The model under review builds one solid part; all positions refer to its coordinate system, in mm. A direction names the side the tool comes from. Coordinates: 2 decimals unless noted, no trailing zeros. Answer in a Markdown table with one row per item.
from build123d import *

# Parameters (mm, degrees)
SKETCH1_W                                        = 80
SKETCH1_H                                        = 50
BOSS_EXTRUDE1_DEPTH                              = 30
CBORE_FOR_M10_HEX_HEAD_BOLT8_D                   = 5
CBORE_FOR_M10_HEX_HEAD_BOLT8_CBORE_D             = 10
CBORE_FOR_M10_HEX_HEAD_BOLT8_CBORE_DEPTH         = 5
CBORE_FOR_M10_HEX_HEAD_BOLT9_D                   = 5
CBORE_FOR_M10_HEX_HEAD_BOLT9_CBORE_D             = 10
CBORE_FOR_M10_HEX_HEAD_BOLT9_CBORE_DEPTH         = 5
CSK_FOR_M10_FLAT_HEAD_MACHINE_SCREW1_D           = 5
CSK_FOR_M10_FLAT_HEAD_MACHINE_SCREW1_CSINK_D     = 10
CSK_FOR_M10_FLAT_HEAD_MACHINE_SCREW1_CSINK_ANGLE = 90


with BuildPart() as part:
    # Sketch1 → Boss-Extrude1 (new body)
    with BuildSketch(Plane.XY):
        with Locations((-9.393939394, -2.727272727)):
            Rectangle(SKETCH1_W, SKETCH1_H)
    extrude(amount=BOSS_EXTRUDE1_DEPTH)

    # CBORE for M10 Hex Head Bolt8 (through all)
    with Locations(Plane.XY.offset(30)):
        with Locations((-29.393939394, 12.272727273)):
            CounterBoreHole(CBORE_FOR_M10_HEX_HEAD_BOLT8_D / 2, CBORE_FOR_M10_HEX_HEAD_BOLT8_CBORE_D / 2, CBORE_FOR_M10_HEX_HEAD_BOLT8_CBORE_DEPTH)

    # CBORE for M10 Hex Head Bolt9 (through all)
    with Locations(Plane.XY.offset(30)):
        with Locations((10.606060606, 2.272727273)):
            CounterBoreHole(CBORE_FOR_M10_HEX_HEAD_BOLT9_D / 2, CBORE_FOR_M10_HEX_HEAD_BOLT9_CBORE_D / 2, CBORE_FOR_M10_HEX_HEAD_BOLT9_CBORE_DEPTH)

    # CSK for M10 Flat Head Machine Screw1 (through all)
    with Locations(Plane.XY.offset(30)):
        with Locations((-9.393939394, -7.727272727)):
            CounterSinkHole(CSK_FOR_M10_FLAT_HEAD_MACHINE_SCREW1_D / 2, CSK_FOR_M10_FLAT_HEAD_MACHINE_SCREW1_CSINK_D / 2, counter_sink_angle=CSK_FOR_M10_FLAT_HEAD_MACHINE_SCREW1_CSINK_ANGLE)


solid = part.part
(1) Machinability: for faces 4 (the cylindrical face through (-30.74, 14.38, 12.32)), 5 (the cylindrical face through (-34.39, 12.49, 27.54)), which of the approach directions +Z, -Z, +X, -X, +Y, -Y give a long, thin tool a straight path to every point of the face, cutting with its end or side? Answer none if there is none.
Report:
| item | result |
|---|---|
| face 4 | +Z, -Z |
| face 5 | +Z |
(2) The part is to be moulded in two halves that separate along X. For faces 1 (the conical face through (-11.89, -6.94, 27.62)), 2 (the flat face through (-49.394, -3, 15)), 3 (the flat face through (30.606, -3, 15)), say which applies: +X half, -X half, draft (parallel to the pull), parting line (faces both ways), or undercut.
Report:
| item | result |
|---|---|
| face 1 | undercut |
| face 2 | -X half |
| face 3 | +X half |
(3) To check wall thickness, follow line 1 (X direction, y = 0, z = 23.5); line 2 (X direction, y = 13.5, z = 25.75). State the ranges of each line that lie inside material, in increasing order. Write a range as [from, to].
Report:
| item | result |
|---|---|
| line 1 | [-49.39, 9.56], [11.65, 30.61] |
| line 2 | [-49.39, -34.24], [-24.55, 30.61] |
(4) Insertion check: P1, Ø6, axis at x = -9.39, y = -7.73, coming from the +Z side. The pin has a flat end and moves straight along its axis. Give the tip position at first contact, or say it passes through.
Report:
| item | result |
|---|---|
| P1 | z = 28 |
